Drawing for the job (mm, zero at the part's lowest x, y, z). Give positions to 0.01 mm unless a question says otherwise; leave off trailing zeros. Order: outer loops, then holes, each group sorted by start corner. A loop starts at its lowest first (then second) coordinate and runs counter-clockwise, first axis right, second up. Notation, with made-up numbers: (77.5, 46) - (87.5, 46) arc R15 ccw to (87.5, 72) - close; hole circle Ø5 at (-28, 49.25). An arc over 180 degrees is marked (long way). One line per item, written item: value.
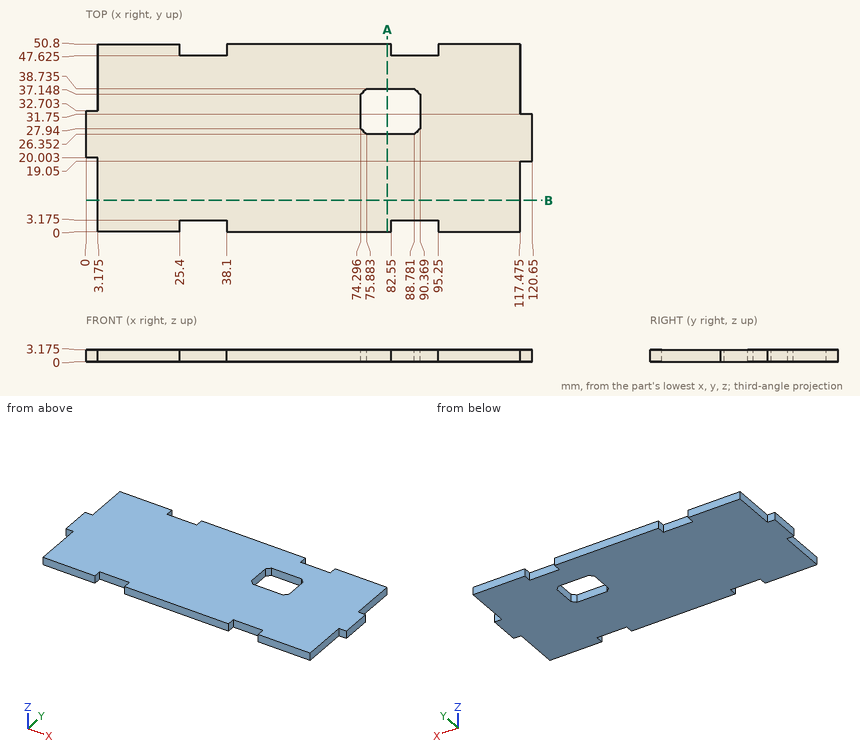
(1) Slice it at B-B, the plane y = 8.5. Give the cut face in (x, z) (1 decimal), and give its area (3 significant figures).
Completed:
outline: (3.2, 0) - (117.5, 0) - (117.5, 3.2) - (3.2, 3.2) - close
area: 363 mm²
(2) Pin check, flat tips, straight feed: P1, Ø1, axis at x = 2, z = 1, coming from the +Y side; P2, Ø1.6, axis at x = 119, z = 2, coming from the -Y side; P3, Ø1, axis at y = 1.5, z = 2, coming from the +X side (1 decimal). Stop position of each tip, or through.
Completed:
P1: y = 32.7
P2: y = 19.05
P3: x = 117.5
(3) Slice it at A-A, the plane x = 81.5. Give the cut face in (y, z) (1 decimal).
Completed:
outline: (0, 0) - (26.4, 0) - (26.4, 3.2) - (0, 3.2) - close; (38.7, 0) - (50.8, 0) - (50.8, 3.2) - (38.7, 3.2) - close
(4) Drill centre lines: line 1 (Y direction, x = 86, z = 2.85) (1 decimal); line 2 (X direction, y = 36.5, z = 1.95) (1 decimal); line 3 (X direction, y = 13.5, z = 2.6) (1 decimal). Where is each one in solid material? Low to high.
Completed:
line 1: 3.2 to 26.4, 38.7 to 47.6
line 2: 3.2 to 74.3, 90.4 to 117.5
line 3: 3.2 to 117.5
